Verification items for the finished model (mm, model axes). Face numbers are marked on the shaded views. A direction names the side the tool comes from. Give positions to 0.01 mm unless a question says otherwise; leave off trailing zeros. Write each loop counter-clockwise with the first axis right and the second up, starting at its lowest first coordinate (ties: lowest second). Pieces come first, ordered by that corner, then holes. Notation, with made-up numbers: (23, 23) -> (43, 23) arc R30 ccw to (43, 59) -> close; hole circle Ø8 at (82, -35). An arc over 180 degrees is marked (long way). Use one line per item in the form item = value. Start each with the question number.
(1) Depth check by flat-ended pin: pin 1 Ø6 at (y, z) = (-9, -23) entering from -X; pin 2 Ø22 at (x, y) = (43.5, 5) entering from -Z; pin 3 Ø5 at (x, y) = (57.5, -18.5) entering from -Z; pin 4 Ø0.8 at (x, y) = (34, 10.5) entering from +Z. Enter the tip coordinate at first touch or a pass-through.
(2) Section check A-A, the plane y = -20. Record the cut outline in (x, z), plus the area to 3 significant figures.
(3) Section check C-C, the plane x = 6. Record the cut outline in (y, z), plus the area to 3 significant figures.
(4) Scan lines: L1, parallel to Y at x = 47, z = -22; L2, parallel to Y at x = 87, z = -13.5; L3, parallel to Z at x = 111.5, y = -18. Record each from-to range of solid material in increasing order.
(5) Section check D-D, the plane z = -4.5. Record the cut outline in (x, y).
(6) Set-up check for the marked faces 4, 5, 6, 7 and 8: record each of +Z, -Z, +X, -X, +Y, -Y from which the full face is reachable in a straight line by a thin tool's end or side.
(7) Section check B-B, the plane x = 83.5. Record the cut outline in (y, z), plus the area to 3 significant figures.
(8) Release check for a two-part mould opening along Z. For the marked faces 1, 2 and 3 record: pulls with the +Z half, pulls with the -Z half, needs draft (parallel to the pull), parting line crosses it, or undercut.
from build123d import *

# Parameters (mm, degrees)
F1_DEPTH  = 167
F3_DEPTH  = 11
F5_DEPTH  = 11
F7_DEPTH  = 152.001
F8_R      = 3
F9_DEPTH  = 78.501
F10_R     = 3
F11_DEPTH = 64.501
F12_R     = 15
F13_DEPTH = 21
F14_R     = 15
F15_DEPTH = 21


with BuildPart() as f1:
    # F0 (on Right) → F1 (new body)
    with BuildSketch(Plane.YZ):
        Polygon((-9, 0), (-25, 0), (-25, -1), (-10, -1), (-10, -15), (0, -15), (10, -15), (10, -1), (25, -1), (25, 0), (9, 0), (9, -14), (0, -14), (-9, -14), align=None)
    extrude(amount=F1_DEPTH)

    # F2 (on Front) → F3 (join, symmetric)
    with BuildSketch(Plane.XZ):
        with BuildLine():
            Line((152, -55), (152, -15))
            Line((152, -15), (105, -15))
            Line((105, -15), (105, -55))
            ThreePointArc((105, -55), (128.5, -78.5), (152, -55))
        make_face()
    extrude(amount=F3_DEPTH, both=True)

    # F4 (on Front) → F5 (join, symmetric)
    with BuildSketch(Plane.XZ):
        Polygon((59, -15), (19, -15), (19, -50), (37, -77), (59, -77), align=None)
    extrude(amount=F5_DEPTH, both=True)

    # F6 (on face) → F7 (cut, through all)
    with BuildSketch(Plane.YZ.offset(152)):
        Polygon((0, -16), (-10, -16), (-10, -83.886804), (0, -83.886804), (10, -83.886804), (10, -16), align=None)
    extrude(amount=-F7_DEPTH, mode=Mode.SUBTRACT)

    # F8 (on face) → F9 (cut, through all)
    with BuildSketch(Plane.XY):
        with Locations((83.5, 20)):
            Circle(F8_R)
        with Locations((83.5, -20)):
            Circle(F8_R)
    extrude(amount=-F9_DEPTH, mode=Mode.SUBTRACT)

    # F10 (on face) → F11 (cut, through all)
    with BuildSketch(Plane.XY.offset(-14)):
        with Locations((161, 0)):
            Circle(F10_R)
        with Locations((6, 0)):
            Circle(F10_R)
    extrude(amount=-F11_DEPTH, mode=Mode.SUBTRACT)

    # F12 (on face) → F13 (join, through all)
    with BuildSketch(Plane.XZ.offset(11)):
        with Locations((128.5, -55)):
            Circle(F12_R)
    extrude(amount=-F13_DEPTH)

    # F14 (on face) → F15 (join, through all)
    with BuildSketch(Plane.XZ.offset(11)):
        with Locations((38.9975, -42)):
            Circle(F14_R)
    extrude(amount=-F15_DEPTH)


solid = f1.part
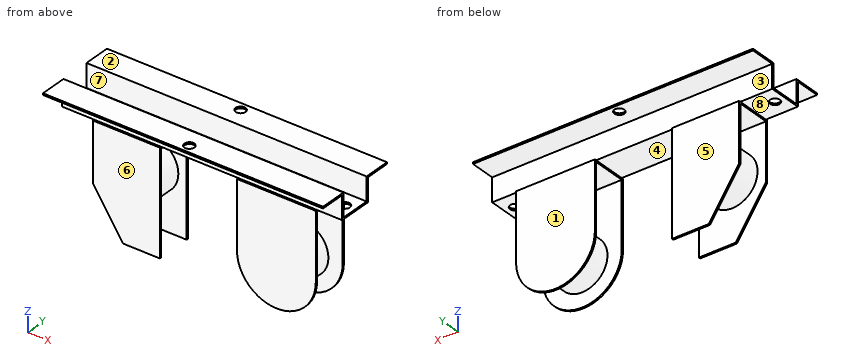
Completed:
q1.pin_1 = 19
q1.pin_2 = -77
q1.pin_3 = -1
q1.pin_4 = 0
q2.outline = (0, -1) -> (80.5, -1) -> (80.5, 0) -> (0, 0) -> close; (86.5, -1) -> (167, -1) -> (167, 0) -> (86.5, 0) -> close
q2.area = 161 mm²
q3.outline = (-25, -1) -> (-10, -1) -> (-10, -15) -> (-3, -15) -> (-3, -14) -> (-9, -14) -> (-9, 0) -> (-25, 0) -> close; (3, -15) -> (10, -15) -> (10, -1) -> (25, -1) -> (25, 0) -> (9, 0) -> (9, -14) -> (3, -14) -> close
q3.area = 72.0 mm²
q4.L1 = -11 to -10, 10 to 11
q4.L2 = -10 to -9, 9 to 10
q4.L3 = -1 to 0
q5.outline = (0, -10) -> (167, -10) -> (167, -9) -> (0, -9) -> close; (0, 9) -> (167, 9) -> (167, 10) -> (0, 10) -> close
q6.face_4 = -Z, +Y, -Y
q6.face_5 = -Z, +X, -X, +Y
q6.face_6 = -Z, +X, -X, -Y
q6.face_7 = +Z, +X, -X
q6.face_8 = -Z, -X, +Y, -Y
q7.outline = (-25, -1) -> (-23, -1) -> (-23, 0) -> (-25, 0) -> close; (-17, -1) -> (-10, -1) -> (-10, -15) -> (10, -15) -> (10, -1) -> (17, -1) -> (17, 0) -> (9, 0) -> (9, -14) -> (-9, -14) -> (-9, 0) -> (-17, 0) -> close; (23, -1) -> (25, -1) -> (25, 0) -> (23, 0) -> close
q7.area = 66.0 mm²
q8.face_1 = needs draft
q8.face_2 = pulls with the +Z half
q8.face_3 = undercut
